from build123d import *

# Parameters (mm, degrees)
SKETCH_1_R                   = 35
EXTRUDE_1_DEPTH              = 2.5
SKETCH_2_R                   = 31.5
EXTRUDE_2_DEPTH              = 2.5
SKETCH_3_R                   = 34
EXTRUDE_3_DEPTH              = 6
HOLE_WIZARD_M4_1_D           = 4.5
HOLE_WIZARD_M4_1_CBORE_D     = 8
HOLE_WIZARD_M4_1_CBORE_DEPTH = 5
HOLE_WIZARD_M4_1_2_D         = 3.3
PATTERN_CIRCULAR_1_COUNT     = 8
PATTERN_CIRCULAR_2_COUNT     = 6
SKETCH_11_W                  = 8
SKETCH_11_H                  = 12
CUT_EXTRUDE_1_DEPTH          = 5
SKETCH_12_W                  = 10
SKETCH_12_H                  = 60
EXTRUDE_4_DEPTH              = 10
SKETCH_13_W                  = 200
SKETCH_13_H                  = 130
CUT_EXTRUDE_2_DEPTH          = 12
PATTERN_CIRCULAR_3_COUNT     = 8
FILLET_1_R                   = 0.1


with BuildPart() as part:
    # 스케치1 → 보스-돌출1 (new body)
    with BuildSketch(Plane(origin=(0, 0, 0), x_dir=(1, 0, 0), z_dir=(0, 1, 0))):
        with BuildLine():
            Line((0, -55), (-65, -55))
            Line((-65, -55), (-65, 55))
            Line((-65, 55), (0, 55))
            ThreePointArc((0, 55), (55, 0), (0, -55))
        make_face()
        Circle(SKETCH_1_R, mode=Mode.SUBTRACT)
    extrude(amount=EXTRUDE_1_DEPTH)

    # 스케치2 → 보스-돌출2 (add)
    with BuildSketch(Plane(origin=(0, 2.5, 0), x_dir=(1, 0, 0), z_dir=(0, 1, 0))):
        with BuildLine():
            Line((-65, 55), (-65, -55))
            Line((-65, -55), (0, -55))
            ThreePointArc((0, -55), (55, 0), (0, 55))
            Line((0, 55), (-65, 55))
        make_face()
        Circle(SKETCH_2_R, mode=Mode.SUBTRACT)
    extrude(amount=EXTRUDE_2_DEPTH)

    # 스케치3 → 보스-돌출3 (add)
    with BuildSketch(Plane(origin=(0, 5, 0), x_dir=(1, 0, 0), z_dir=(0, 1, 0))):
        with BuildLine():
            Line((-65, 55), (-65, -55))
            Line((-65, -55), (0, -55))
            ThreePointArc((0, -55), (55, 0), (0, 55))
            Line((0, 55), (-65, 55))
        make_face()
        Circle(SKETCH_3_R, mode=Mode.SUBTRACT)
    extrude(amount=EXTRUDE_3_DEPTH)

    # Hole Wizard M4 _ _ _ _ _ _1 (through all)
    with Locations(Plane(origin=(0, 11, 0), x_dir=(1, 0, 0), z_dir=(0, 1, 0))):
        with Locations((0, 49)):
            hole_wizard_m4_1 = CounterBoreHole(HOLE_WIZARD_M4_1_D / 2, HOLE_WIZARD_M4_1_CBORE_D / 2, HOLE_WIZARD_M4_1_CBORE_DEPTH)

    # Hole Wizard M4 _ _ _ _1 2 (through all)
    with Locations(Plane(origin=(0, 11, 0), x_dir=(1, 0, 0), z_dir=(0, 1, 0))):
        with Locations((0, 39)):
            hole_wizard_m4_1_2 = Hole(HOLE_WIZARD_M4_1_2_D / 2)

    # 원형 패턴1: Hole Wizard M4 _ _ _ _ _ _1 ×8 about axis
    pattern_circular_1_axis = Axis((0, 0, 0), (0, 1, 0))
    for i in range(1, PATTERN_CIRCULAR_1_COUNT):
        add(hole_wizard_m4_1.rotate(pattern_circular_1_axis, i * 360 / PATTERN_CIRCULAR_1_COUNT), mode=Mode.SUBTRACT)

    # 원형 패턴2: Hole Wizard M4 _ _ _ _1 2 ×6 about axis
    pattern_circular_2_axis = Axis((0, 0, 0), (0, 1, 0))
    for i in range(1, PATTERN_CIRCULAR_2_COUNT):
        add(hole_wizard_m4_1_2.rotate(pattern_circular_2_axis, i * 360 / PATTERN_CIRCULAR_2_COUNT), mode=Mode.SUBTRACT)

    # 스케치11 → 컷-돌출1 (cut, symmetric)
    with BuildSketch(Plane(origin=(0, 11, 0), x_dir=(1, 0, 0), z_dir=(0, 1, 0))):
        with Locations((0, 55)):
            Rectangle(SKETCH_11_W, SKETCH_11_H)
    cut_extrude_1 = extrude(amount=CUT_EXTRUDE_1_DEPTH, both=True, mode=Mode.SUBTRACT)

    # 스케치12 → 보스-돌출4 (add)
    with BuildSketch(Plane(origin=(0, 11, 0), x_dir=(1, 0, 0), z_dir=(0, 1, 0))):
        with Locations((-60, 0)):
            Rectangle(SKETCH_12_W, SKETCH_12_H)
    extrude(amount=EXTRUDE_4_DEPTH)

    # 스케치13 → 컷-돌출2 (cut, through all)
    with BuildSketch(Plane(origin=(0, 11, 0), x_dir=(1, 0, 0), z_dir=(0, 1, 0))):
        Rectangle(SKETCH_13_W, SKETCH_13_H)
        with BuildLine():
            Line((-65, -30), (-46.097722286, -30))
            ThreePointArc((-46.097722286, -30), (55, 0), (-46.097722286, 30))
            Line((-46.097722286, 30), (-65, 30))
            Line((-65, 30), (-65, -30))
        make_face(mode=Mode.SUBTRACT)
    extrude(amount=-CUT_EXTRUDE_2_DEPTH, mode=Mode.SUBTRACT)

    # 원형 패턴3: 컷-돌출1 ×8 about axis, 1 skipped
    pattern_circular_3_axis = Axis((0, 0, 0), (0, 1, 0))
    add([cut_extrude_1.rotate(pattern_circular_3_axis, i * 360 / PATTERN_CIRCULAR_3_COUNT) for i in range(1, PATTERN_CIRCULAR_3_COUNT) if i not in (2,)], mode=Mode.SUBTRACT)

    # 필렛1
    fillet_1_edges = [part.edges().sort_by_distance(p)[0] for p in [
        (-35, 2.5, 0),
        (-34, 5, 0),
    ]]
    fillet(fillet_1_edges, radius=FILLET_1_R)


solid = part.part
Here's how the part is built. I have some questions about the finished solid (model axes, mm). A direction names the side the tool comes from. Coordinates: 2 decimals unless noted, no trailing zeros. Order: outer loops, then holes, each group sorted by start corner. A loop starts at its lowest first (then second) coordinate and runs counter-clockwise, first axis right, second up. Notation, with made-up numbers: M 29.5,26 L 43.5,26 A25 cw 43.5,39 Z; hole C -22.5,50.5 d11. An arc over 180 degrees is marked long. Answer as CSV lines item,"result". Start each with the question number.
1. On a 3-axis mill with a long thin cutter (end or side, diameter ignored), from which of +Z, -Z, +X, -X, +Y, -Y can I reach the whole of each face in a straight line? I mean faces 4 (the cylindrical face through (0, 9, -45)), 5 (the flat face through (-33.861, 8.535, 39.518)), 6 (the flat face through (-25, 11, 24)), 7 (the cylindrical face through (-31.76, 8.54, 31.88)), 8 (the flat face through (-4, 9, 52)). Say none if no direction works.
2. I need wall thicknesses on line 1 (X direction, y = 7.3, z = 0); line 2 (Z direction, x = 0, y = 7.25); line 3 (Z direction, x = 31, y = 9.5). Which ranges of each line are inside material? Lowest first, please. Write a range as [from, to].
3. We'd pull the mould along X, two halves only. Please class faces 1 (the flat face through (-55, 16, 0)), 2 (the cylindrical face through (18.28, 8.01, -28.67)), 3 (the flat face through (52, 6, 0)): released by +X, released by -X, zero draft, split by the parting line, or undercut.
4. I want a section at B-B, the plane z = 0. Count the separate pieces of the cut face and the enclosed holes in it, and give its area (3 significant figures).
5. I want a section at C-C, the plane y = 14.75. Write out the boundary of the cut face in (x, z), and give its area (3 significant figures).
6. For pin 1 (12 mm diameter, centred on x = -38.5, z = -37.5, fed in from +Y); pin 2 (8 mm diameter, centred on y = 7, z = -36, fed in from -X); pin 3 (5 mm diameter, centred on x = 0, z = 49, fed in from +Y); pin 4 (4 mm diameter, centred on x = 34.65, z = -34.65, fed in from +Y), each with a flat end and sliding along its axis, tell me the tip position at first contact or that it passes through.
7. I want a section at A-A, the plane x = -49. Write out the boundary of the cut face in (y, z), and give its area (3 significant figures).
Recorded:
1,face 4,"-Z, +Y"
1,face 5,"-X, +Y"
1,face 6,"+Z, -Z, +X, +Y"
1,face 7,"+Y"
1,face 8,"+Z, +Y"
2,line 1,"x = [-65, -53], [-45, -34], [34, 45]"
2,line 2,"z = [-45, -40.65], [-37.35, -34], [34, 37.35], [40.65, 45]"
2,line 3,"z = [-45.43, -36.29], [-33.01, -13.96], [13.96, 33.01], [36.29, 45.43]"
3,face 1,"released by +X"
3,face 2,"undercut"
3,face 3,"zero draft"
4,separate pieces,"4"
4,enclosed holes,"0"
4,area,"536 mm2"
5,outline,"M -65,-30 L -55,-30 L -55,30 L -65,30 Z"
5,area,"600 mm2"
6,pin 1,"stops at y = 11"
6,pin 2,"stops at x = -44.73"
6,pin 3,"stops at y = 6"
6,pin 4,"passes through"
7,outline,"M 0,-30 L 11,-30 L 11,-4 L 6,-4 L 6,-2.25 L 0,-2.25 Z; M 0,2.25 L 6,2.25 L 6,4 L 11,4 L 11,30 L 0,30 Z"
7,area,"593 mm2"
